```python
from build123d import *

# Parameters (mm, degrees)
SKETCH_1_W      = 22.5
SKETCH_1_H      = 12.5
EXTRUDE_1_DEPTH = 28
SKETCH_2_W      = 32
SKETCH_2_H      = 12.5
EXTRUDE_2_DEPTH = 2
SKETCH_3_R      = 3.388656212
EXTRUDE_3_DEPTH = 2.5
SKETCH_4_R      = 1
EXTRUDE_4_DEPTH = 2


with BuildPart() as part:
    # 草图1 → 凸台-拉伸1 (new body)
    with BuildSketch(Plane.XY):
        Rectangle(SKETCH_1_W, SKETCH_1_H)
    extrude(amount=EXTRUDE_1_DEPTH)

    # 草图2 → 凸台-拉伸2 (add)
    with BuildSketch(Plane.XY.offset(28)):
        Rectangle(SKETCH_2_W, SKETCH_2_H)
    extrude(amount=EXTRUDE_2_DEPTH)

    # 草图3 → 凸台-拉伸3 (add)
    with BuildSketch(Plane.XY.offset(30)):
        with Locations(Location((4.874315739, 0, 0), (0, 0, 180))):
            Circle(SKETCH_3_R)
    extrude(amount=EXTRUDE_3_DEPTH)

    # 草图4 → 凸台-拉伸4 (add)
    with BuildSketch(Plane.XY.offset(32.5)):
        with Locations((4.874315739, 0)):
            Circle(SKETCH_4_R)
    extrude(amount=EXTRUDE_4_DEPTH)


solid = part.part
```
Geometry check sheet. Reference: the model listing, model coordinates, mm. A direction names the side the tool comes from. Coordinates: 2 decimals unless noted, no trailing zeros. Write each loop counter-clockwise with the first axis right and the second up, starting at its lowest first coordinate (ties: lowest second). Pieces come first, ordered by that corner, then holes. Notation, with made-up numbers: M 13,72.25 L 65,72.25 A32 ccw 65,107.25 Z; hole C 54,53 d3. An arc over 180 degrees is marked long. Use one line per item in the form item = value. Start each with the question number.
1) Section check B-B on x = 0. Enter the section's corners in (y, z), and give its area (3 significant figures).
2) Go/stop test with flat-tipped pins: pin 1 Ø5 at (x, y) = (9, -4) entering from +Z; pin 2 Ø5 at (x, y) = (-13.5, -1.5) entering from -Z; pin 3 Ø6 at (y, z) = (0.5, 10) entering from +X; pin 4 Ø5 at (x, y) = (-8, 2.5) entering from +Z. Record where each tip stops, or that it passes through.
3) Section check D-D on y = 0. Enter the section's corners in (x, z), and give its area (3 significant figures).
4) Set-up check for faces 1 (the flat face through (-11.25, 0, 14)), 2 (the flat face through (4, -1, 32.5)), 3 (the flat face through (11.25, 0, 14)): record each of +Z, -Z, +X, -X, +Y, -Y from which the full face is reachable in a straight line by a thin tool's end or side.
5) Thickness scan on probe 1 along X at (y, z) = (-3, 24); probe 2 along Z at (x, y) = (13.5, 5.75); probe 3 along Z at (x, y) = (9, 3). Record the ranges inside material, lowest first. Write a range as from..to.
6) Section check C-C on z = 25.5. Enter the section's corners in (x, y).
7) Section check A-A on y = 4.25. Enter the section's corners in (x, z), and give its area (3 significant figures).
Responses:
q1.outline = M -6.25,0 L 6.25,0 L 6.25,30 L -6.25,30 Z
q1.area = 375 mm2
q2.pin_1 = 32.5
q2.pin_2 = 0
q2.pin_3 = 11.25
q2.pin_4 = 30
q3.outline = M -16,28 L -11.25,28 L -11.25,0 L 11.25,0 L 11.25,28 L 16,28 L 16,30 L 8.26,30 L 8.26,32.5 L 5.87,32.5 L 5.87,34.5 L 3.87,34.5 L 3.87,32.5 L 1.49,32.5 L 1.49,30 L -16,30 Z
q3.area = 715 mm2
q4.face_1 = -Z, -X, +Y, -Y
q4.face_2 = +Z
q4.face_3 = -Z, +X, +Y, -Y
q5.probe_1 = -11.25..11.25
q5.probe_2 = 28..30
q5.probe_3 = 0..30
q6.outline = M -11.25,-6.25 L 11.25,-6.25 L 11.25,6.25 L -11.25,6.25 Z
q7.outline = M -16,28 L -11.25,28 L -11.25,0 L 11.25,0 L 11.25,28 L 16,28 L 16,30 L -16,30 Z
q7.area = 694 mm2
